```python
from build123d import *

# Parameters (mm, degrees)
F0_W      = 203.2
F0_H      = 330.2
F1_DEPTH  = 254
F2_T      = -2.54
F4_DEPTH  = 25.4
F6_DEPTH  = 25.4
F8_DEPTH  = 222.25
F10_DEPTH = 222.25
F11_W     = 203.2
F11_H     = 3.175
F12_DEPTH = 38.1
F13_W     = 203.2
F13_H     = 3.175
F14_DEPTH = 38.1
F15_R     = 5.08
F16_DEPTH = 25.4
F17_R     = 3.175
F18_R     = 9.525


with BuildPart() as f1:
    # F0 (on Top) → F1 (new body)
    with BuildSketch(Plane.XY):
        Rectangle(F0_W, F0_H)
    extrude(amount=F1_DEPTH)

    # F2
    f2_openings = [f1.faces().sort_by_distance(p)[0] for p in [
        (0, 0, 0),
    ]]
    offset(amount=F2_T, openings=f2_openings)

    # F3 (on face) → F4 (cut)
    with BuildSketch(Plane.XZ.offset(165.1)):
        with BuildLine():
            Line((-25.4, 0), (0, 0))
            Line((0, 0), (0, 127))
            ThreePointArc((0, 127), (-17.9605122421, 134.4394877579), (-25.4, 152.4))
            Line((-25.4, 152.4), (-25.4, 0))
        make_face()
        with BuildLine():
            Line((0, 127), (0, 0))
            Line((0, 0), (25.4, 0))
            Line((25.4, 0), (25.4, 152.4))
            ThreePointArc((25.4, 152.4), (17.9605122421, 134.4394877579), (0, 127))
        make_face()
        with BuildLine():
            ThreePointArc((-25.4, 152.4), (-17.9605122421, 134.4394877579), (0, 127))
            Line((0, 127), (0, 152.4))
            Line((0, 152.4), (-25.4, 152.4))
        make_face()
        with BuildLine():
            Line((0, 152.4), (0, 127))
            ThreePointArc((0, 127), (17.9605122421, 134.4394877579), (25.4, 152.4))
            Line((25.4, 152.4), (0, 152.4))
        make_face()
        with BuildLine():
            Line((-25.4, 152.4), (0, 152.4))
            Line((0, 152.4), (25.4, 152.4))
            ThreePointArc((25.4, 152.4), (0, 177.8), (-25.4, 152.4))
        make_face()
    extrude(amount=-F4_DEPTH, mode=Mode.SUBTRACT)

    # F5 (on face) → F6 (cut)
    with BuildSketch(Plane(origin=(0, 165.1, 0), x_dir=(-1, 0, 0), z_dir=(0, 1, 0))):
        with BuildLine():
            Line((-38.1, 0), (0, 0))
            Line((0, 0), (0, 114.3))
            ThreePointArc((0, 114.3), (-26.9407683632, 125.4592316368), (-38.1, 152.4))
            Line((-38.1, 152.4), (-38.1, 0))
        make_face()
        with BuildLine():
            Line((0, 114.3), (0, 0))
            Line((0, 0), (38.1, 0))
            Line((38.1, 0), (38.1, 152.4))
            ThreePointArc((38.1, 152.4), (26.9407683632, 125.4592316368), (0, 114.3))
        make_face()
        with BuildLine():
            ThreePointArc((-38.1, 152.4), (-26.9407683632, 125.4592316368), (0, 114.3))
            Line((0, 114.3), (0, 152.4))
            Line((0, 152.4), (-38.1, 152.4))
        make_face()
        with BuildLine():
            Line((0, 152.4), (0, 114.3))
            ThreePointArc((0, 114.3), (26.9407683632, 125.4592316368), (38.1, 152.4))
            Line((38.1, 152.4), (0, 152.4))
        make_face()
        with BuildLine():
            Line((-38.1, 152.4), (0, 152.4))
            Line((0, 152.4), (38.1, 152.4))
            ThreePointArc((38.1, 152.4), (0, 190.5), (-38.1, 152.4))
        make_face()
    extrude(amount=-F6_DEPTH, mode=Mode.SUBTRACT)

    # F7 (on face) → F8 (join)
    with BuildSketch(Plane(origin=(0, 0, 0), x_dir=(1, 0, 0), z_dir=(0, 0, -1))):
        Polygon((99.06, 101.6), (99.06, 0), (99.06, -101.6), (101.6, -101.6), (101.6, 101.6), align=None)
    extrude(amount=F8_DEPTH)

    # F9 (on face) → F10 (join)
    with BuildSketch(Plane(origin=(0, 0, 0), x_dir=(1, 0, 0), z_dir=(0, 0, -1))):
        Polygon((-99.06, -101.6), (-99.06, 0), (-99.06, 101.6), (-101.6, 101.6), (-101.6, -101.6), align=None)
    extrude(amount=F10_DEPTH)

    # F11 (on face) → F12 (join)
    with BuildSketch(Plane.YZ.offset(101.6)):
        with Locations((0, -220.6625)):
            Rectangle(F11_W, F11_H)
    extrude(amount=F12_DEPTH)

    # F13 (on face) → F14 (join)
    with BuildSketch(Plane(origin=(-101.6, 0, 0), x_dir=(0, -1, 0), z_dir=(-1, 0, 0))):
        with Locations((0, -220.6625)):
            Rectangle(F13_W, F13_H)
    extrude(amount=F14_DEPTH)

    # F15 (on face) → F16 (cut)
    with BuildSketch(Plane(origin=(0, 0, -222.25), x_dir=(1, 0, 0), z_dir=(0, 0, -1))):
        with Locations((120.65, 76.2)):
            Circle(F15_R)
        with Locations((120.65, -76.2)):
            Circle(F15_R)
        with Locations((-120.65, 76.2)):
            Circle(F15_R)
        with Locations((-120.65, -76.2)):
            Circle(F15_R)
    extrude(amount=-F16_DEPTH, mode=Mode.SUBTRACT)

    # F17
    f17_edges = [f1.edges().sort_by_distance(p)[0] for p in [
        (101.6, 0, -219.075),
        (99.06, 0, -222.25),
        (-99.06, 0, -222.25),
        (-101.6, 0, -219.075),
        (-101.6, -165.1, 127),
        (0, -165.1, 254),
        (101.6, -165.1, 127),
        (-101.6, 165.1, 127),
        (0, 165.1, 254),
        (101.6, 165.1, 127),
        (-101.6, 0, 254),
        (101.6, 0, 254),
    ]]
    fillet(f17_edges, radius=F17_R)

    # F18
    f18_edges = [f1.edges().sort_by_distance(p)[0] for p in [
        (-139.7, 101.6, -220.6625),
        (-139.7, -101.6, -220.6625),
        (139.7, -101.6, -220.6625),
        (139.7, 101.6, -220.6625),
    ]]
    fillet(f18_edges, radius=F18_R)


solid = f1.part
```
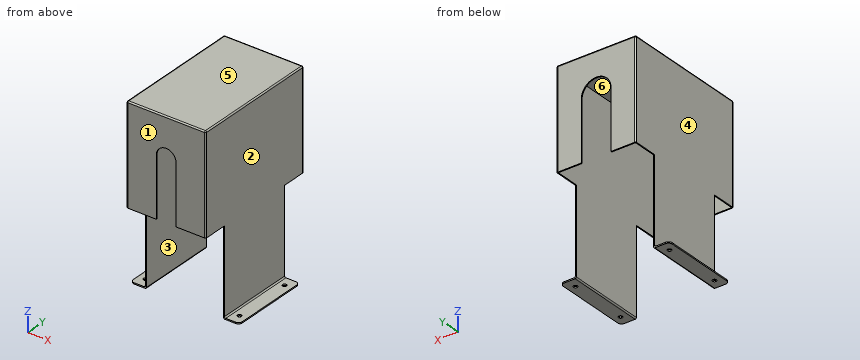
The model under review builds one solid part; all positions refer to its coordinate system, in mm. Face numbers are marked on the shaded views. A direction names the side the tool comes from. Coordinates: 2 decimals unless noted, no trailing zeros. Write each loop counter-clockwise with the first axis right and the second up, starting at its lowest first coordinate (ties: lowest second). Pieces come first, ordered by that corner, then holes. Notation, with made-up numbers: (76.25, 49.25) -> (131.25, 49.25) arc R27 cw to (131.25, 72.25) -> close; hole circle Ø7 at (10.5, 53.25). An arc over 180 degrees is marked (long way). One line per item, written item: value. Start each with the question number.
Q1. Add section D-D, the plane z = 220. Give the boundary of the cut face in (x, y) (3 decimals).
Q2. Add section A-A, the plane z = 136. Give the boundary of the cut face in (x, y) (3 decimals).
Q3. The part is to be moulded in two halves that separate along X. For the marked faces 1, 2, 3 and 4, say which applies: +X half, -X half, draft (parallel to the pull), parting line (faces both ways), or undercut.
Q4. To check wall thickness, follow probe 1 along Y at (x, z) = (120.65, -220.35); probe 2 along X at (y, z) = (76.2, -219.8); probe 3 along X at (y, z) = (-93.5, -143). State the ranges of each line that lie inside material, in increasing order.
Q5. Add section B-B, the plane x = -90.5. Give the boundary of the cut face in (y, z) (3 decimals), then the cut area to 3 significant figures.
Q6. For the marked faces 5 and 6, list the 3-axis set-ups (+Z, -Z, +X, -X, +Y, -Y) from which the entire face can be reached by the end or side of a thin tool; tool diameter is ignored.
Q7. Clearance check with flat-ended pins moving along their axes: P1, Ø2, axis at y = 163.5, z = 103, coming from the +X side; P2, Ø8, axis at x = -120.65, y = -76.2, coming from the +Z side; P3, Ø19, axis at x = -53.5, y = -145.5, coming from the -Z side; P4, Ø17.5, axis at x = 127, y = 32, coming from the +Z side (3 decimals). State where each tip first meets the part, or that it passes through.
Q8. Add section C-C, the plane y = -119. Give the boundary of the cut face in (x, z) (3 decimals), then the cut area to 3 significant figures.
Response:
1. outline: (-101.6, -161.925) arc R3.175 ccw to (-98.425, -165.1) -> (98.425, -165.1) arc R3.175 ccw to (101.6, -161.925) -> (101.6, 161.925) arc R3.175 ccw to (98.425, 165.1) -> (-98.425, 165.1) arc R3.175 ccw to (-101.6, 161.925) -> close; hole (-99.06, -162.56) -> (99.06, -162.56) -> (99.06, 162.56) -> (-99.06, 162.56) -> close
2. outline: (-101.6, -161.925) arc R3.175 ccw to (-98.425, -165.1) -> (-25.4, -165.1) -> (-25.4, -162.56) -> (-99.06, -162.56) -> (-99.06, 162.56) -> (-38.1, 162.56) -> (-38.1, 165.1) -> (-98.425, 165.1) arc R3.175 ccw to (-101.6, 161.925) -> close; (25.4, -165.1) -> (98.425, -165.1) arc R3.175 ccw to (101.6, -161.925) -> (101.6, 161.925) arc R3.175 ccw to (98.425, 165.1) -> (38.1, 165.1) -> (38.1, 162.56) -> (99.06, 162.56) -> (99.06, -162.56) -> (25.4, -162.56) -> close
3. face 1: draft
3. face 2: +X half
3. face 3: undercut
3. face 4: -X half
4. probe 1: -101.6 to -81.28, -71.12 to 71.12, 81.28 to 101.6
4. probe 2: -139.7 to -125.73, -115.57 to -99.14, 99.14 to 115.57, 125.73 to 139.7
4. probe 3: -101.6 to -99.06, 99.06 to 101.6
5. outline: (-165.1, 0) -> (-162.56, 0) -> (-162.56, 251.46) -> (162.56, 251.46) -> (162.56, 0) -> (165.1, 0) -> (165.1, 250.825) arc R3.175 ccw to (161.925, 254) -> (-161.925, 254) arc R3.175 ccw to (-165.1, 250.825) -> close
5. area: 2,110 mm²
6. face 5: +Z, +X, -X, +Y, -Y
6. face 6: -Z
7. P1: x = 101.55
7. P2: through
7. P3: z = 251.46
7. P4: z = -219.075
8. outline: (-101.6, 0) -> (-99.06, 0) -> (-99.06, 251.46) -> (99.06, 251.46) -> (99.06, 0) -> (101.6, 0) -> (101.6, 250.825) arc R3.175 ccw to (98.425, 254) -> (-98.425, 254) arc R3.175 ccw to (-101.6, 250.825) -> close
8. area: 1,790 mm²
